Here's how the part is built. I have some questions about the finished solid (model axes, mm). Round coordinates to 2 decimals unless told otherwise and drop trailing zeros. Write each loop counter-clockwise with the first axis right and the second up, starting at its lowest first coordinate (ties: lowest second). Pieces come first, ordered by that corner, then holes. Notation, with made-up numbers: (-11.75, 37.25) -> (32.25, 37.25) arc R11 cw to (32.25, 56.25) -> close; hole circle Ø8 at (-28.5, -13.5). An arc over 180 degrees is marked (long way). Put each result on its own line as item: value. Start each with the question number.
1) I want a section at C-C, the plane z = 42. List the corners of the cut face in (x, y) for me, then the cut area to 3 significant figures.
2) I want a section at B-B, the plane z = 10. List the corners of the cut face in (x, y) for me, then the cut area to 3 significant figures.
3) I want a section at A-A, the plane y = 5.25. List the corners of the cut face in (x, z) for me, then the cut area to 3 significant figures.
4) Will these pins go through, and if not, where does the flat tip stop? P1, Ø7.5, axis at x = 0, z = 22.5, coming from the -Y side; P2, Ø3, axis at x = 6.5, z = 47, coming from the +Y side; P3, Ø5, axis at x = -34.5, z = 85, coming from the +Y side; P4, Ø6, axis at x = 0, z = 80, coming from the -Y side.
5) I want a section at D-D, the plane x = -21.5. List the corners of the cut face in (y, z) for me, then the cut area to 3 significant figures.
6) If I drill on line 1 along Z through (x, y) = (-33.75, 4.5); line 2 along Z through (x, y) = (-33.75, 0.9); line 3 along X through (y, z) = (6.5, 8.75), over which ranges is the centre line in solid material (lowest first)? Write a range as [from, to].
from build123d import *

# Parameters (mm, degrees)
SKETCH_1_W          = 95
SKETCH_1_H          = 95
SKETCH_1_R          = 3.2
EXTRUDE_1_DEPTH     = 10
SKETCH_2_R          = 5.25
CUT_EXTRUDE_1_DEPTH = 7
FILLET_1_R          = 10
SKETCH_3_R          = 3.25
CUT_EXTRUDE_2_DEPTH = 10
SKETCH_4_W          = 10.4
SKETCH_4_H          = 10.4
SKETCH_4_R          = 3.25
CUT_EXTRUDE_3_DEPTH = 7
SKETCH_5_W          = 1
SKETCH_5_H          = 5
EXTRUDE_2_DEPTH     = 0.5


with BuildPart() as part:
    # 스케치1 → 보스-돌출1 (new body)
    with BuildSketch(Plane(origin=(0, 0, 0), x_dir=(1, 0, 0), z_dir=(0, 1, 0))):
        with Locations((3.75, -46.25)):
            Rectangle(SKETCH_1_W, SKETCH_1_H)
        with Locations((16.25, -8.75)):
            Circle(SKETCH_1_R, mode=Mode.SUBTRACT)
        with Locations((-33.75, -8.75)):
            Circle(SKETCH_1_R, mode=Mode.SUBTRACT)
        with Locations((41.25, -8.75)):
            Circle(SKETCH_1_R, mode=Mode.SUBTRACT)
        with Locations((-33.75, -83.75)):
            Circle(SKETCH_1_R, mode=Mode.SUBTRACT)
        with Locations((41.25, -83.75)):
            Circle(SKETCH_1_R, mode=Mode.SUBTRACT)
    extrude(amount=EXTRUDE_1_DEPTH)

    # 스케치2 → 컷-돌출1 (cut)
    with BuildSketch(Plane(origin=(0, 10, 0), x_dir=(1, 0, 0), z_dir=(0, 1, 0))):
        with Locations((16.25, -8.75)):
            Circle(SKETCH_2_R)
        with Locations((-33.75, -8.75)):
            Circle(SKETCH_2_R)
        with Locations((41.25, -8.75)):
            Circle(SKETCH_2_R)
        with Locations((41.25, -83.75)):
            Circle(SKETCH_2_R)
        with Locations((-33.75, -83.75)):
            Circle(SKETCH_2_R)
    extrude(amount=-CUT_EXTRUDE_1_DEPTH, mode=Mode.SUBTRACT)

    # 필렛1
    fillet_1_edges = [part.edges().sort_by_distance(p)[0] for p in [
        (51.25, 5, -1.25),
        (51.25, 5, 93.75),
        (-43.75, 5, 93.75),
        (-43.75, 5, -1.25),
    ]]
    fillet(fillet_1_edges, radius=FILLET_1_R)

    # 스케치3 → 컷-돌출2 (cut)
    with BuildSketch(Plane(origin=(0, 10, 0), x_dir=(1, 0, 0), z_dir=(0, 1, 0))):
        with Locations((0, -22.5)):
            Circle(SKETCH_3_R)
        with Locations((0, -80)):
            Circle(SKETCH_3_R)
    extrude(amount=-CUT_EXTRUDE_2_DEPTH, mode=Mode.SUBTRACT)

    # 스케치4 → 컷-돌출3 (cut)
    with BuildSketch(Plane.XZ):
        with Locations((0, 22.5)):
            Rectangle(SKETCH_4_W, SKETCH_4_H)
        with Locations((0, 22.5)):
            Circle(SKETCH_4_R, mode=Mode.SUBTRACT)
        with Locations((0, 80)):
            Rectangle(SKETCH_4_W, SKETCH_4_H)
        with Locations((0, 80)):
            Circle(SKETCH_4_R, mode=Mode.SUBTRACT)
    extrude(amount=-CUT_EXTRUDE_3_DEPTH, mode=Mode.SUBTRACT)

    # 스케치5 → 보스-돌출2 (add)
    with BuildSketch(Plane(origin=(0, 10, 0), x_dir=(1, 0, 0), z_dir=(0, 1, 0))):
        with Locations((0, -91.25)):
            Rectangle(SKETCH_5_W, SKETCH_5_H)
    extrude(amount=EXTRUDE_2_DEPTH)


solid = part.part
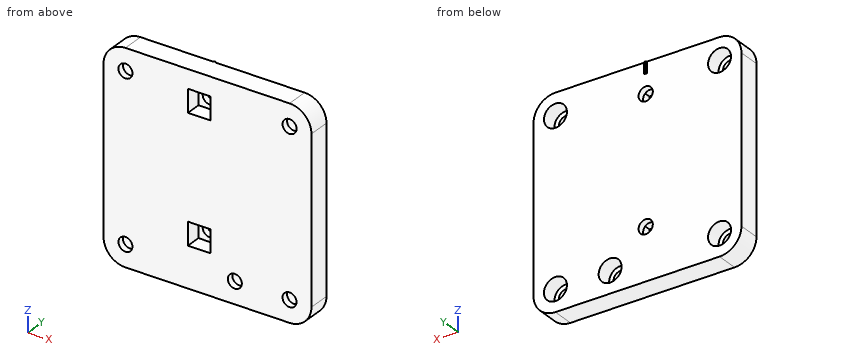
Findings:
1. outline: (-43.75, 0) -> (51.25, 0) -> (51.25, 10) -> (-43.75, 10) -> close
1. area: 950 mm2
2. outline: (-43.75, 0) -> (-36.7, 0) -> (-36.7, 3) -> (-38.85, 3) -> (-38.85, 10) -> (-43.75, 10) -> close; (-30.8, 0) -> (13.3, 0) -> (13.3, 3) -> (11.15, 3) -> (11.15, 10) -> (-28.65, 10) -> (-28.65, 3) -> (-30.8, 3) -> close; (19.2, 0) -> (38.3, 0) -> (38.3, 3) -> (36.15, 3) -> (36.15, 10) -> (21.35, 10) -> (21.35, 3) -> (19.2, 3) -> close; (44.2, 0) -> (51.25, 0) -> (51.25, 10) -> (46.35, 10) -> (46.35, 3) -> (44.2, 3) -> close
2. area: 683 mm2
3. outline: (-43.75, 8.75) arc R10 ccw to (-33.75, -1.25) -> (41.25, -1.25) arc R10 ccw to (51.25, 8.75) -> (51.25, 83.75) arc R10 ccw to (41.25, 93.75) -> (-33.75, 93.75) arc R10 ccw to (-43.75, 83.75) -> close; hole circle Ø10.5 at (-33.75, 8.75); hole circle Ø10.5 at (-33.75, 83.75); hole (-5.2, 17.3) -> (5.2, 17.3) -> (5.2, 27.7) -> (-5.2, 27.7) -> close; hole (-5.2, 74.8) -> (5.2, 74.8) -> (5.2, 85.2) -> (-5.2, 85.2) -> close; hole circle Ø10.5 at (16.25, 8.75); hole circle Ø10.5 at (41.25, 8.75); hole circle Ø10.5 at (41.25, 83.75)
3. area: 8,290 mm2
4. P1: stops at y = 7
4. P2: stops at y = 10
4. P3: stops at y = 3
4. P4: passes through
5. outline: (0, -1.25) -> (10, -1.25) -> (10, 93.75) -> (0, 93.75) -> close
5. area: 950 mm2
6. line 1: z = [-1.25, 3.5], [14, 78.5], [89, 93.75]
6. line 2: z = [-1.25, 5.55], [11.95, 80.55], [86.95, 93.75]
6. line 3: x = [-43.75, -39], [-28.5, 11], [21.5, 36], [46.5, 51.25]
